Geometry check sheet. Reference: the model listing, model coordinates, mm. A direction names the side the tool comes from. Give positions to 0.01 mm unless a question says otherwise; leave off trailing zeros. Order: outer loops, then holes, each group sorted by start corner. A loop starts at its lowest first (then second) coordinate and runs counter-clockwise, first axis right, second up. Notation, with made-up numbers: M 37.25,4.5 L 41.25,4.5 A14 ccw 41.25,19.5 Z; hole C 63.25,-36.5 d2. An arc over 180 degrees is marked long. Answer as CSV lines item,"result". Start each with the question number.
Q1. Thickness scan on line 1 (Z direction, x = 54, y = 61); line 2 (Y direction, x = 17, z = 223.5); line 3 (X direction, y = 62, z = 229). Record the ranges inside material, lowest first.
Q2. Section check A-A, the plane y = 29.5. Record the boundary of the cut face in (x, z), then the cut area to 3 significant figures.
Q3. Go/stop test with flat-tipped pins: pin 1 (10 mm diameter, centred on y = 50, z = 189, fed in from -X); pin 2 (3 mm diameter, centred on x = 47, y = 27.5, fed in from -Z); pin 3 (1.7 mm diameter, centred on x = 62, y = 28, fed in from +Z); pin 4 (12 mm diameter, centred on x = 48.5, y = 36, fed in from -Z). Record where each tip stops, or that it passes through.
Q4. Section check C-C, the plane x = 37. Record the boundary of the cut face in (y, z), then the cut area to 3 significant figures.
Q5. Section check B-B, the plane y = 42. Record the boundary of the cut face in (x, z).
Q6. Mould release check, pull along X, two halves, no side actions. Record for faces 5 (the flat face through (-1, 60, 123)), 6 (the flat face through (-43.5, 30, 104)), 7 (the flat face through (57, 63, 119.72)), 8 (the flat face through (49.5, 48, 103)): +X half, -X half, draft (parallel to the pull), parting line (faces both ways), or undercut.
Q7. Section check D-D, the plane z = 44. Record the boundary of the cut face in (x, y).
Q8. Set-up check for faces 1 (the flat face through (-49.5, 50, 103)), 2 (the flat face through (-47, 30, 100.25)), 3 (the flat face through (62, 30, 187)), 4 (the flat face through (85, 61, 29.72)): record each of +Z, -Z, +X, -X, +Y, -Y from which the full face is reachable in a straight line by a thin tool's end or side.
```python
from build123d import *

# Parameters (mm, degrees)
SKETCH1_W             = 6
SKETCH1_H             = 8
BOSS_EXTRUDE1_DEPTH   = 60
SKETCH1_W_2           = 5.75
SKETCH1_H_2           = 10
BOSS_EXTRUDE1_2_DEPTH = 60
BOSS_EXTRUDE1_3_DEPTH = 60
BOSS_EXTRUDE1_4_DEPTH = 60
BOSS_EXTRUDE2_DEPTH   = 6
BOSS_EXTRUDE3_DEPTH   = 24


with BuildPart() as part:
    # Sketch1 → Boss-Extrude1 (new body)
    with BuildSketch(Plane(origin=(0, 0, 0), x_dir=(1, 0, 0), z_dir=(0, 1, 0))):
        with Locations((-46.5, -104.25)):
            Rectangle(SKETCH1_W, SKETCH1_H)
    extrude(amount=BOSS_EXTRUDE1_DEPTH)



with BuildPart() as body_2:
    # Sketch1 → Boss-Extrude1 2 (new body)
    with BuildSketch(Plane(origin=(0, 0, 0), x_dir=(1, 0, 0), z_dir=(0, 1, 0))):
        with Locations((-62.125, -182)):
            Rectangle(SKETCH1_W_2, SKETCH1_H_2)
    extrude(amount=BOSS_EXTRUDE1_2_DEPTH)


with BuildPart() as body_3:
    # Sketch1 → Boss-Extrude1 3 (new body)
    with BuildSketch(Plane(origin=(0, 0, 0), x_dir=(1, 0, 0), z_dir=(0, 1, 0))):
        with Locations((62.125, -182)):
            Rectangle(SKETCH1_W_2, SKETCH1_H_2)
    extrude(amount=BOSS_EXTRUDE1_3_DEPTH)


with BuildPart() as body_4:
    # Sketch1 → Boss-Extrude1 4 (new body)
    with BuildSketch(Plane(origin=(0, 0, 0), x_dir=(1, 0, 0), z_dir=(0, 1, 0))):
        with Locations((46.5, -104.25)):
            Rectangle(SKETCH1_W, SKETCH1_H)
    extrude(amount=BOSS_EXTRUDE1_4_DEPTH)


with BuildPart() as part_1:
    add(part.part)

    add(body_2.part)  # Boss-Extrude2 merges body 2

    add(body_3.part)  # Boss-Extrude2 merges body 3

    add(body_4.part)  # Boss-Extrude2 merges body 4
    # Sketch2 → Boss-Extrude2 (add)
    with BuildSketch(Plane(origin=(0, 60, 0), x_dir=(1, 0, 0), z_dir=(0, 1, 0))):
        Polygon((-52.5, -119.720396317), (-62, -119.720396317), (-65, -122.720396317), (-65, -244.720396317), (65, -244.720396317), (65, -122.720396317), (62, -119.720396317), (52.5, -119.720396317), (49.5, -116.720396317), (49.5, -32.720396317), (52.5, -29.720396317), (97.407038705, -29.720396317), (63.440871486, 0), (-63.440871486, 0), (-97.407038705, -29.720396317), (-52.5, -29.720396317), (-49.5, -32.720396317), (-49.5, -116.720396317), align=None)
    extrude(amount=BOSS_EXTRUDE2_DEPTH)

    # Sketch4 → Boss-Extrude3 (add)
    with BuildSketch(Plane.XZ.offset(-60)):
        Polygon((89.81407741, 29.720396317), (61.562195905, 5), (-61.562195905, 5), (-89.81407741, 29.720396317), (-97.407038705, 29.720396317), (-63.440871486, 0), (63.440871486, 0), (97.407038705, 29.720396317), align=None)
    extrude(amount=BOSS_EXTRUDE3_DEPTH)


solid = part_1.part
```
Answer block:
1,line 1,"z = 0 to 29.72, 119.72 to 244.72"
1,line 2,"y = 60 to 66"
1,line 3,"x = -65 to 65"
2,outline,"M -65,177 L -59.25,177 L -59.25,187 L -65,187 Z; M -49.5,100.25 L -43.5,100.25 L -43.5,108.25 L -49.5,108.25 Z; M 43.5,100.25 L 49.5,100.25 L 49.5,108.25 L 43.5,108.25 Z; M 59.25,177 L 65,177 L 65,187 L 59.25,187 Z"
2,area,"211 mm2"
3,pin 1,"stops at x = -65"
3,pin 2,"stops at z = 100.25"
3,pin 3,"stops at z = 187"
3,pin 4,"stops at z = 0"
4,outline,"M 36,0 L 66,0 L 66,244.72 L 60,244.72 L 60,5 L 36,5 Z"
4,area,"1,590 mm2"
5,outline,"M -97.41,29.72 L -63.44,0 L 63.44,0 L 97.41,29.72 L 89.81,29.72 L 61.56,5 L -61.56,5 L -89.81,29.72 Z; M -65,177 L -59.25,177 L -59.25,187 L -65,187 Z; M -49.5,100.25 L -43.5,100.25 L -43.5,108.25 L -49.5,108.25 Z; M 43.5,100.25 L 49.5,100.25 L 49.5,108.25 L 43.5,108.25 Z; M 59.25,177 L 65,177 L 65,187 L 59.25,187 Z"
6,face 5,"undercut"
6,face 6,"undercut"
6,face 7,"draft"
6,face 8,"+X half"
7,outline,"M -49.5,60 L 49.5,60 L 49.5,66 L -49.5,66 Z"
8,face 1,"-X, +Y, -Y"
8,face 2,"+X, -X, -Y"
8,face 3,"+Z, +X, -X, -Y"
8,face 4,"+X, +Y, -Y"
